```python
from build123d import *

# Parameters (mm, degrees)
ESBO_O2_W                  = 273.42
ESBO_O2_H                  = 221.24
RESSALTO_EXTRUS_O1_DEPTH   = 80
ESBO_O3_W                  = 267.42
ESBO_O3_H                  = 215.24
CORTE_EXTRUS_O1_DEPTH      = 80
ESBO_O4_W                  = 59.55
ESBO_O4_H                  = 29.05
CORTE_EXTRUS_O3_DEPTH      = 194.200436076
ESBO_O5_W                  = 59.55
ESBO_O5_H                  = 29.05
CORTE_EXTRUS_O4_DEPTH      = 194.200436076
CORTE_EXTRUS_O5_DEPTH      = 194.200436076
CORTE_EXTRUS_O5_DEPTH_BACK = 194.200436076
ESBO_O6_W                  = 59.55
ESBO_O6_H                  = 29.05
CORTE_EXTRUS_O6_DEPTH      = 194.200436076
CORTE_EXTRUS_O6_DEPTH_BACK = 194.200436076
ESBO_O7_R                  = 2.7
ESBO_O8_R                  = 2.7
CORTE_EXTRUS_O7_DEPTH      = 194.200436076
ESBO_O9_R                  = 2.7
CORTE_EXTRUS_O8_DEPTH      = 194.200436076


with BuildPart() as part:
    # Esboço2 → Ressalto-extrusão1 (new body)
    with BuildSketch(Plane.XY):
        Rectangle(ESBO_O2_W, ESBO_O2_H)
    extrude(amount=RESSALTO_EXTRUS_O1_DEPTH)

    # Esboço3 → Corte-extrusão1 (cut)
    with BuildSketch(Plane.XY):
        Rectangle(ESBO_O3_W, ESBO_O3_H)
    extrude(amount=CORTE_EXTRUS_O1_DEPTH, mode=Mode.SUBTRACT)

    # Esboço4 → Corte-extrusão3 (cut, through all)
    with BuildSketch(Plane(origin=(0, 0, 0), x_dir=(0, 0, -1), z_dir=(1, 0, 0))):
        with Locations((-39.439615286, 0)):
            Rectangle(ESBO_O4_W, ESBO_O4_H)
    extrude(amount=CORTE_EXTRUS_O3_DEPTH, mode=Mode.SUBTRACT)

    # Esboço5 → Corte-extrusão4 (cut, through all)
    with BuildSketch(Plane(origin=(0, 0, 0), x_dir=(0, 0, -1), z_dir=(1, 0, 0))):
        with Locations((-40, 71.095)):
            Rectangle(ESBO_O5_W, ESBO_O5_H)
        with Locations((-40, -71.095)):
            Rectangle(ESBO_O5_W, ESBO_O5_H)
    extrude(amount=-CORTE_EXTRUS_O4_DEPTH, mode=Mode.SUBTRACT)

    # Esboço6 → Corte-extrusão5 (cut, two sides: drawn at the far end of the back side and taken through both)
    with BuildSketch(Plane(origin=(0, 0, 0), x_dir=(1, 0, 0), z_dir=(0, 1, 0)).offset(-CORTE_EXTRUS_O5_DEPTH_BACK)):
        with Locations((71.935, -40)):
            Rectangle(ESBO_O6_W, ESBO_O6_H)
    extrude(amount=CORTE_EXTRUS_O5_DEPTH + CORTE_EXTRUS_O5_DEPTH_BACK, mode=Mode.SUBTRACT)

    # Esboço7 → Corte-extrusão6 (cut, two sides: drawn at the far end of the back side and taken through both)
    with BuildSketch(Plane(origin=(0, 0, 0), x_dir=(1, 0, 0), z_dir=(0, 1, 0)).offset(-CORTE_EXTRUS_O6_DEPTH_BACK)):
        with Locations(Location((91.21, -22.675, 0), (0, 0, 270))):
            Circle(ESBO_O7_R)
        with Locations(Location((69.21, -22.675, 0), (0, 0, 270))):
            Circle(ESBO_O7_R)
        with Locations(Location((47.21, -22.675, 0), (0, 0, 270))):
            Circle(ESBO_O7_R)
        with Locations(Location((91.21, -57.325, 0), (0, 0, 270))):
            Circle(ESBO_O7_R)
        with Locations(Location((69.21, -57.325, 0), (0, 0, 270))):
            Circle(ESBO_O7_R)
        with Locations(Location((47.21, -57.325, 0), (0, 0, 270))):
            Circle(ESBO_O7_R)
        with Locations(Location((39.36, -28.975, 0), (0, 0, 270))):
            Circle(ESBO_O7_R)
        with Locations(Location((39.36, -51.025, 0), (0, 0, 270))):
            Circle(ESBO_O7_R)
    extrude(amount=CORTE_EXTRUS_O6_DEPTH + CORTE_EXTRUS_O6_DEPTH_BACK, mode=Mode.SUBTRACT)

    # Esboço8 → Corte-extrusão7 (cut, through all)
    with BuildSketch(Plane(origin=(0, 0, 0), x_dir=(0, 0, -1), z_dir=(1, 0, 0))):
        with Locations((-59.275, -88.42)):
            Circle(ESBO_O8_R)
        with Locations((-37.275, -88.42)):
            Circle(ESBO_O8_R)
        with Locations((-15.275, -88.42)):
            Circle(ESBO_O8_R)
        with Locations((-15.275, -53.77)):
            Circle(ESBO_O8_R)
        with Locations((-37.275, -53.77)):
            Circle(ESBO_O8_R)
        with Locations((-59.275, -53.77)):
            Circle(ESBO_O8_R)
        with Locations((-7.425, -82.12)):
            Circle(ESBO_O8_R)
        with Locations((-7.425, -60.07)):
            Circle(ESBO_O8_R)
        with Locations((-59.275, 53.77)):
            Circle(ESBO_O8_R)
        with Locations((-37.275, 53.77)):
            Circle(ESBO_O8_R)
        with Locations((-15.275, 53.77)):
            Circle(ESBO_O8_R)
        with Locations((-7.425, 60.07)):
            Circle(ESBO_O8_R)
        with Locations((-7.425, 82.12)):
            Circle(ESBO_O8_R)
        with Locations((-15.275, 88.42)):
            Circle(ESBO_O8_R)
        with Locations((-37.275, 88.42)):
            Circle(ESBO_O8_R)
        with Locations((-59.275, 88.42)):
            Circle(ESBO_O8_R)
    extrude(amount=-CORTE_EXTRUS_O7_DEPTH, mode=Mode.SUBTRACT)

    # Esboço9 → Corte-extrusão8 (cut, through all)
    with BuildSketch(Plane(origin=(0, 0, 0), x_dir=(0, 0, -1), z_dir=(1, 0, 0))):
        with Locations(Location((-58.714615286, 17.325, 0), (0, 0, 180))):
            Circle(ESBO_O9_R)
        with Locations(Location((-36.714615286, 17.325, 0), (0, 0, 180))):
            Circle(ESBO_O9_R)
        with Locations(Location((-14.714615286, 17.325, 0), (0, 0, 180))):
            Circle(ESBO_O9_R)
        with Locations(Location((-14.714615286, -17.325, 0), (0, 0, 180))):
            Circle(ESBO_O9_R)
        with Locations(Location((-36.714615286, -17.325, 0), (0, 0, 180))):
            Circle(ESBO_O9_R)
        with Locations(Location((-58.714615286, -17.325, 0), (0, 0, 180))):
            Circle(ESBO_O9_R)
        with Locations(Location((-6.864615286, 11.025, 0), (0, 0, 180))):
            Circle(ESBO_O9_R)
        with Locations(Location((-6.864615286, -11.025, 0), (0, 0, 180))):
            Circle(ESBO_O9_R)
    extrude(amount=CORTE_EXTRUS_O8_DEPTH, mode=Mode.SUBTRACT)


solid = part.part
```
Verification items for the finished model (mm, model axes). A direction names the side the tool comes from. Coordinates: 2 decimals unless noted, no trailing zeros. Order: outer loops, then holes, each group sorted by start corner. A loop starts at its lowest first (then second) coordinate and runs counter-clockwise, first axis right, second up. Notation, with made-up numbers: (37.25, 74) - (83.25, 74) arc R17 cw to (83.25, 105) - close; hole circle Ø9 at (74.25, -29). An arc over 180 degrees is marked (long way). Return JSON: item names as keys, results as strings.
(1) Section check A-A, the plane x = 13.5. Record the cut outline in (y, z).
Filled sheet:
{"outline": "(-110.62, 0) - (-107.62, 0) - (-107.62, 80) - (-110.62, 80) - close; (107.62, 0) - (110.62, 0) - (110.62, 80) - (107.62, 80) - close"}
(2) Mould release check, pull along X, two halves, no side actions. Record for faces 1 (the flat face through (133.71, -25, 39)), 2 (the flat face through (-2, 107.62, 39)), 3 (the flat face through (-2, -110.62, 39)), 4 (the flat face through (136.71, 23, 39)): pulls with the +X half, pulls with the -X half, needs draft (parallel to the pull), parting line crosses it, or undercut.
Filled sheet:
{"face 1": "undercut", "face 2": "undercut", "face 3": "needs draft", "face 4": "pulls with the +X half"}
(3) Access from +Z, -Z, +X, -X, +Y, -Y to the whole of each face (thin tool, end or side, straight path). Record for faces 5 (the flat face through (-133.71, -2, 39)), 6 (the flat face through (-2, 110.62, 39)).
Filled sheet:
{"face 5": "+Z, -Z", "face 6": "+Z, -Z, +X, -X, +Y"}
(4) Thickness scan on line 1 along X through (y, z) = (-15, 64.5); line 2 along Y through (x, z) = (-107.5, 55); line 3 along X through (y, z) = (-76.5, 24.5). Record the ranges inside material, lowest first.
Filled sheet:
{"line 1": "x = -136.71 to -133.71, 133.71 to 136.71", "line 2": "y = -110.62 to -107.62, 107.62 to 110.62", "line 3": "x = 133.71 to 136.71"}
(5) Section check B-B, the plane y = -96.5. Record the cut outline in (x, z), and give its area (3 significant figures).
Filled sheet:
{"outline": "(-136.71, 0) - (-133.71, 0) - (-133.71, 80) - (-136.71, 80) - close; (133.71, 0) - (136.71, 0) - (136.71, 80) - (133.71, 80) - close", "area": "480 mm^2"}
(6) Go/stop test with a flat-tipped pin: pin 1 (3 mm diameter, centred on y = 80.5, z = 56, fed in from -X). Record where the tip stops, or that it passes through.
Filled sheet:
{"pin 1": "stops at x = 133.71"}
